Input: part model. Units: mm. Frame: model coordinates. A direction names the side the tool comes from. Give positions to 0.01 mm unless a question says otherwise; leave off trailing zeros. Loops run counter-clockwise (first coordinate to the right, second up) from the corner with the lowest first, then second, coordinate; pieces in that order, holes last. Notation, with made-up numbers: (78, 58.5) - (120, 58.5) arc R23 ccw to (120, 85.5) - close; hole circle Ø5 at (34.5, 39). An arc over 180 degrees is marked (long way). One line per question, with ' | ' between items. Start each with the question number.
from build123d import *

# Parameters (mm, degrees)
BROCA_DE_ROSQUEAR_PARA_TARRAXA_DE_M5X0_8_D     = 4.2
BROCA_DE_ROSQUEAR_PARA_TARRAXA_DE_M5X0_8_DEPTH = 7
BROCA_DE_ROSQUEAR_PARA_TARRAXA_DE_M5X0_8_TIP   = 1.2618073


with BuildPart() as part:
    # Esboço2 → Revolução1 (revolve)
    with BuildSketch(Plane(origin=(0, 0, 0), x_dir=(1, 0, 0), z_dir=(0, 1, 0))):
        with BuildLine():
            Line((-66.33, 2), (-70, 2))
            Line((-70, 2), (-70, 4.4))
            Line((-70, 4.4), (-32, 4.4))
            Line((-32, 4.4), (-32, -2))
            Line((-32, -2), (-34.76, -2))
            ThreePointArc((-34.76, -2), (-36.07, -0.842172747), (-37.38, -2))
            Line((-37.38, -2), (-50, -2))
            Line((-50, -2), (-50, -6))
            Line((-50, -6), (-60, -6))
            Line((-60, -6), (-60, 2))
            Line((-60, 2), (-63.33, 2))
            ThreePointArc((-63.33, 2), (-64.83, 3.5), (-66.33, 2))
        make_face()
    revolve(axis=Axis((0, 0, -4.826033988), (0, 0, 1)))

    # Broca de rosquear para tarraxa de M5x0.81
    with Locations(Plane.XY.offset(6)):
        with Locations((-27.5, 47.631397208), (27.5, 47.631397208), (55, 0), (27.5, -47.631397208), (-27.5, -47.631397208), (-55, 0)):
            Hole(BROCA_DE_ROSQUEAR_PARA_TARRAXA_DE_M5X0_8_D / 2, depth=BROCA_DE_ROSQUEAR_PARA_TARRAXA_DE_M5X0_8_DEPTH)
            with Locations((0, 0, -(BROCA_DE_ROSQUEAR_PARA_TARRAXA_DE_M5X0_8_DEPTH + BROCA_DE_ROSQUEAR_PARA_TARRAXA_DE_M5X0_8_TIP / 2))):  # 118° drill point
                Cone(0, BROCA_DE_ROSQUEAR_PARA_TARRAXA_DE_M5X0_8_D / 2, BROCA_DE_ROSQUEAR_PARA_TARRAXA_DE_M5X0_8_TIP, mode=Mode.SUBTRACT)


solid = part.part
Q1. First-contact query: pin 1 (1 mm diameter, centred on y = 54, z = 4, fed in from -X); pin 2 (2 mm diameter, centred on x = -11, y = -41.5, fed in from +Z); pin 3 (3.5 mm diameter, centred on x = -55, y = 0, fed in from +Z). Flat tips, straight axial feed; report the tip coordinate or a pass-through.
Q2. Line query: L1, parallel to Y at x = 38, z = -2.75; L2, parallel to Y at x = 29.5, z = -2.25; L3, parallel to Y at x = 27.5, z = 1.25. Output: solid intervals per line, ascending. Write a range as from..to.
Q3. Draft query along X for faces 1 (the face through (59.94, -2.64, 1.94)), 2 (the face through (53.06, -0.8, 2.45)), 3 (the face through (52, -42, -2)). Return one class per face: +X half, -X half, draft (parallel to the pull), parting line (faces both ways), or undercut.
Q4. Section A-A, the plane z = 4.25. Output: boundary loops of the cut face in (x, y), plus the area to 3 significant figures.
Q5. Access query for faces 4 (the face through (-56.94, -0.8, 2.45)), 5 (the face through (-45, -23, 6)). Directions: +Z, -Z, +X, -X, +Y, -Y. A direction counts if a zero-diameter tool reaches every point of the face in a straight line with its end or side. Return the directions, or none.
Solved:
1) pin 1: stops at x = -27.16 | pin 2: stops at z = 2 | pin 3: stops at z = -1.21
2) L1: y = -58.79..-54.12, -50.91..50.91, 54.12..58.79 | L2: y = -63.48..-59.39, -56.06..-12.4, 12.4..56.06, 59.39..63.48 | L3: y = -53.33..-49.73, -45.53..-24.79, -21.84..-16.36, 16.36..21.84, 24.79..45.53, 49.73..53.33
3) face 1: parting line | face 2: undercut | face 3: draft
4) outline: circle Ø120 at (0, 0); hole circle Ø4.2 at (-55, 0); hole circle Ø100 at (0, 0); hole circle Ø4.2 at (-27.5, -47.63); hole circle Ø4.2 at (-27.5, 47.63); hole circle Ø4.2 at (27.5, -47.63); hole circle Ø4.2 at (27.5, 47.63); hole circle Ø4.2 at (55, 0) | area: 3,370 mm²
5) face 4: +Z | face 5: +Z, +X, -X, +Y, -Y
